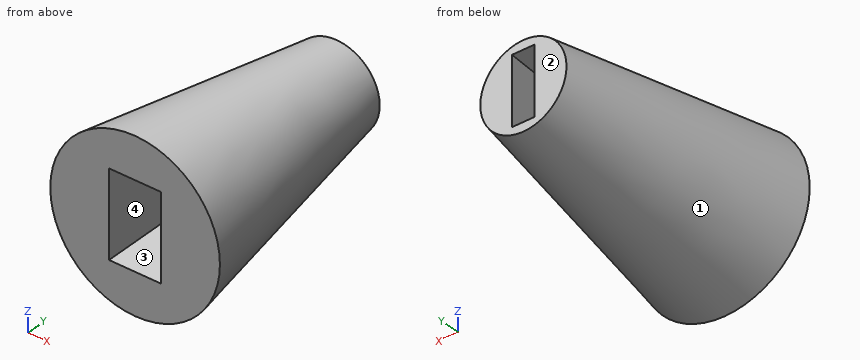
```python
from build123d import *

# Parameters (mm, degrees)
SKETCH_2_R          = 9.5
SKETCH_1_R          = 18.7
SKETCH_5_W          = 11.5
SKETCH_5_H          = 19
CUT_EXTRUDE_1_DEPTH = 32
SKETCH_9_W          = 11.5
SKETCH_9_H          = 19
SKETCH_6_W          = 5
SKETCH_6_H          = 15


with BuildPart() as part:
    # 스케치2 → 로프트1 section 0
    with BuildSketch(Plane(origin=(0, 55, 0), x_dir=(1, 0, 0), z_dir=(0, 1, 0))):
        Circle(SKETCH_2_R)
    # 스케치1 → 로프트1 section 1
    with BuildSketch(Plane(origin=(0, 0, 0), x_dir=(1, 0, 0), z_dir=(0, 1, 0))):
        Circle(SKETCH_1_R)
    loft()

    # 스케치5 → 컷-돌출1 (cut)
    with BuildSketch(Plane.XZ):
        Rectangle(SKETCH_5_W, SKETCH_5_H)
    extrude(amount=-CUT_EXTRUDE_1_DEPTH, mode=Mode.SUBTRACT)

    # 스케치9 → 컷-로프트2 section 0
    with BuildSketch(Plane.XZ.offset(-32)):
        Rectangle(SKETCH_9_W, SKETCH_9_H)
    # 스케치6 → 컷-로프트2 section 1
    with BuildSketch(Plane(origin=(0, 55, 0), x_dir=(1, 0, 0), z_dir=(0, 1, 0))):
        Rectangle(SKETCH_6_W, SKETCH_6_H)
    loft(mode=Mode.SUBTRACT)


solid = part.part
```
The model under review builds one solid part; all positions refer to its coordinate system, in mm. Face numbers are marked on the shaded views. Give positions to 0.01 mm unless a question says otherwise; leave off trailing zeros. Write each loop counter-clockwise with the first axis right and the second up, starting at its lowest first coordinate (ties: lowest second). Pieces come first, ordered by that corner, then holes. Notation, with made-up numbers: (56.5, -7.5) - (91.5, -7.5) arc R16 ccw to (91.5, 7.5) - close; hole circle Ø1 at (31, -21.5). An arc over 180 degrees is marked (long way). Answer in a Markdown table with one row per item. Add a question column.
1. Insertion check: P1, Ø21, axis at y = 20.5, z = -2.5, coming from the -X side; P2, Ø1, axis at x = 1, y = 12, coming from the +Z side; P3, Ø1.5, axis at y = 48.5, z = -7, coming from the -X side; P4, Ø1, axis at x = 1.5, z = 4.5, coming from the +Y side. Each pin has a flat end and moves straight along its axis. Give the tip position at first contact, or say it passes through.
2. Wall thickness on line 1 along Z through (x, y) = (2.5, 45); line 2 along Z through (x, y) = (2.5, 32); line 3 along X through (y, z) = (12.5, 9): over which ranges is each line inside the solid? List them lowest first. Write a range as [from, to].
3. We need section A-A on y = 6. Write out the cut boundary in (x, z).
4. We need section B-B on y = 24.5. Write out the cut boundary in (x, z).
5. Draft analysis for pull direction X (two halves, no side actions). For the marked faces 1, 2, 3 and 4, state which applies: +X half, -X half, draft (parallel to the pull), parting line (faces both ways), or undercut.
Ans:
| question | item | result |
|---|---|---|
| 1 | P1 | stops at x = -16.99 |
| 1 | P2 | stops at z = 16.75 |
| 1 | P3 | stops at x = -8.57 |
| 1 | P4 | passes through |
| 2 | line 1 | z = [-10.89, -8.37], [8.37, 10.89] |
| 2 | line 2 | z = [-13.11, -9.5], [9.5, 13.11] |
| 2 | line 3 | x = [-13.96, -5.75], [5.75, 13.96] |
| 3 | outline | circle Ø35.39 at (0, 0); hole (-5.75, -9.5) - (5.75, -9.5) - (5.75, 9.5) - (-5.75, 9.5) - close |
| 4 | outline | circle Ø29.2 at (0, 0); hole (-5.75, -9.5) - (5.75, -9.5) - (5.75, 9.5) - (-5.75, 9.5) - close |
| 5 | face 1 | parting line |
| 5 | face 2 | draft |
| 5 | face 3 | undercut |
| 5 | face 4 | undercut |
